Geometry check sheet. Reference: the model listing, model coordinates, mm. A direction names the side the tool comes from. Round coordinates to 2 decimals unless told otherwise and drop trailing zeros. Loops run counter-clockwise (first coordinate to the right, second up) from the corner with the lowest first, then second, coordinate; pieces in that order, holes last. Notation, with made-up numbers: M -33,89 L -17,89 A31 ccw -17,113 Z; hole C 29,32 d2. An arc over 180 degrees is marked long. Use one line per item in the form item = value. Start each with the question number.
1. Go/stop test with flat-tipped pins: pin 1 (0.9 mm diameter, centred on x = -41.5, y = 1, fed in from -Z); pin 2 (0.9 mm diameter, centred on x = -42, y = 1, fed in from +Z); pin 3 (1.5 mm diameter, centred on y = 1, z = -4, fed in from +X). Record where each tip stops, or that it passes through.
2. Set-up check for faces 1 (the flat face through (-9.867, 1, 4)), 2 (the flat face through (-41, 1, -7)), 3 (the flat face through (-8, 1, -10)), 4 (the flat face through (-41, 1, -10)): record each of +Z, -Z, +X, -X, +Y, -Y from which the full face is reachable in a straight line by a thin tool's end or side.
3. Material ranges on line 1 (X direction, y = 1.5, z = -3.5); line 2 (X direction, y = 2.4, z = -4.75); line 3 (Z direction, x = -35, y = 1.1), recorded low to high.
4. Cross-section at C-C (z = 4.25). Record the boundary of the cut face in (x, y), then the cut area to 3 significant figures.
5. Draft check along X on faces 5 (the flat face through (-8, 1, 0)), 6 (the flat face through (-39.867, 1, 5)), 7 (the cylindrical face through (-13.48, 1.48, -2.93)). Enter one of: pulls with the +X half, pulls with the -X half, needs draft (parallel to the pull), parting line crosses it, or undercut.
6. Cross-section at A-A (z = -3.5). Record the boundary of the cut face in (x, y), then the cut area to 3 significant figures.
7. Cross-section at B-B (y = 0.6). Record the boundary of the cut face in (x, z).
```python
from build123d import *

# Parameters (mm, degrees)
SKETCH1_R           = 1.5
BOSS_EXTRUDE1_DEPTH = 3


with BuildPart() as part:
    # Sketch1 → Boss-Extrude1 (new body)
    with BuildSketch(Plane(origin=(0, 0, 0), x_dir=(1, 0, 0), z_dir=(0, 1, 0))):
        Polygon((-42.867412192, 7), (-42.867412192, 10), (-39.867412192, 10), (-39.867412192, 13), (-9.867412192, 13), (-9.867412192, 10), (-6.867412192, 10), (-6.867412192, 7), (-9.867412192, 7), (-9.867412192, 0), (-6.867412192, 0), (-6.867412192, -3), (-9.867412192, -3), (-9.867412192, -6), (-39.867412192, -6), (-39.867412192, -3), (-42.867412192, -3), (-42.867412192, 0), (-39.867412192, 0), (-39.867412192, 7), align=None)
        with Locations((-34.867412192, 3.5)):
            Circle(SKETCH1_R, mode=Mode.SUBTRACT)
        with Locations((-14.867412192, 3.5)):
            Circle(SKETCH1_R, mode=Mode.SUBTRACT)
    extrude(amount=BOSS_EXTRUDE1_DEPTH)


solid = part.part
```
Reported:
q1.pin_1 = -10
q1.pin_2 = 3
q1.pin_3 = -9.87
q2.face_1 = +Z, +X, +Y, -Y
q2.face_2 = -X, +Y, -Y
q2.face_3 = -Z, +X, +Y, -Y
q2.face_4 = -Z, -X, +Y, -Y
q3.line_1 = -39.87 to -36.37, -33.37 to -16.37, -13.37 to -9.87
q3.line_2 = -39.87 to -35.7, -34.04 to -15.7, -14.04 to -9.87
q3.line_3 = -13 to -4.99, -2.01 to 6
q4.outline = M -39.87,0 L -9.87,0 L -9.87,3 L -39.87,3 Z
q4.area = 90.0 mm²
q5.face_5 = needs draft
q5.face_6 = pulls with the -X half
q5.face_7 = undercut
q6.outline = M -39.87,0 L -36.37,0 L -36.37,3 L -39.87,3 Z; M -33.37,0 L -16.37,0 L -16.37,3 L -33.37,3 Z; M -13.37,0 L -9.87,0 L -9.87,3 L -13.37,3 Z
q6.area = 72.0 mm²
q7.outline = M -42.87,-10 L -39.87,-10 L -39.87,-13 L -9.87,-13 L -9.87,-10 L -6.87,-10 L -6.87,-7 L -9.87,-7 L -9.87,0 L -6.87,0 L -6.87,3 L -9.87,3 L -9.87,6 L -39.87,6 L -39.87,3 L -42.87,3 L -42.87,0 L -39.87,0 L -39.87,-7 L -42.87,-7 Z; hole C -34.87,-3.5 d3; hole C -14.87,-3.5 d3
